from build123d import *

# Parameters (mm, degrees)
F1_DEPTH = 63.5
F0_W     = 25.4
F0_H     = 19.05
F2_DEPTH = 25.4
F3_DEPTH = 7.9375
F5_R     = 6.35


with BuildPart() as f1:
    # F0 (on Front) → F1 (new body, symmetric)
    with BuildSketch(Plane.XZ):
        Polygon((-41.275, 9.525), (-41.275, -9.525), (41.275, -9.525), (41.275, 9.525), (22.225, 9.525), align=None)
    extrude(amount=F1_DEPTH, both=True)

    # F0 (on Front) → F2 (join, symmetric)
    with BuildSketch(Plane.XZ):
        with BuildLine():
            Line((22.225, 9.525), (41.275, 9.525))
            Line((41.275, 9.525), (41.275, 27.0002))
            ThreePointArc((41.275, 27.0002), (45.9246798487, 38.2255201513), (57.15, 42.8752))
            Line((57.15, 42.8752), (60.325, 42.8752))
            Line((60.325, 42.8752), (60.325, 61.9252))
            Line((60.325, 61.9252), (57.15, 61.9252))
            ThreePointArc((57.15, 61.9252), (32.4542956671, 51.6959043329), (22.225, 27.0002))
            Line((22.225, 27.0002), (22.225, 9.525))
        make_face()
        with Locations((73.025, 52.4002)):
            Rectangle(F0_W, F0_H)
    extrude(amount=F2_DEPTH, both=True)

    # F0 (on Front) → F3 (join, symmetric)
    with BuildSketch(Plane.XZ):
        with BuildLine():
            add(Edge.make_bspline(
                [(-41.275, 9.525), (-41.1149449646, 36.8104875088), (6.9761793129, 62.6372024417), (57.15, 61.9252)],
                knots=[0, 0, 0, 0, 111.5045361635, 111.5045361635, 111.5045361635, 111.5045361635], degree=3))
            Line((-41.275, 9.525), (22.225, 9.525))
            Line((22.225, 9.525), (22.225, 27.0002))
            ThreePointArc((22.225, 27.0002), (32.4542956671, 51.6959043329), (57.15, 61.9252))
        make_face()
    extrude(amount=F3_DEPTH, both=True)

    # F0 (on Front) → F4 (revolve)
    with BuildSketch(Plane.XZ):
        Polygon((85.725, 66.675), (85.725, 61.9252), (85.725, 42.8752), (85.725, 38.1), (111.125, 38.1), (111.125, 66.675), align=None)
    revolve(axis=Axis((85.725, 0, 52.3875), (0, 0, 1)))

    # F5
    f5_edges = [f1.edges().sort_by_distance(p)[0] for p in [
        (-41.275, -63.5, 0),
        (41.275, -63.5, 0),
        (41.275, 63.5, 0),
        (41.275, 0, -9.525),
        (-41.275, 63.5, 0),
    ]]
    fillet(f5_edges, radius=F5_R)


solid = f1.part
Input: part model. Units: mm. Frame: model coordinates. A direction names the side the tool comes from. Round coordinates to 2 decimals unless told otherwise and drop trailing zeros. Order: outer loops, then holes, each group sorted by start corner. A loop starts at its lowest first (then second) coordinate and runs counter-clockwise, first axis right, second up. Notation, with made-up numbers: (68.25, 17.5) - (112.25, 17.5) arc R27 ccw to (112.25, 40.5) - close; hole circle Ø2 at (50, 47.5). An arc over 180 degrees is marked (long way). Use a Markdown table: item, result.
1. Mould query, pull axis X, two halves, no side actions, for faces 1 (the face through (-41.275, -1, 0)), 2 (the face through (86, 0, 38.1)), 3 (the face through (60, 2, 42.875)). Classes: +X half, -X half, draft (parallel to the pull), parting line (faces both ways), or undercut.
Evaluation:
| item | result |
|---|---|
| face 1 | -X half |
| face 2 | draft |
| face 3 | undercut |
2. Access query for faces 4 (the face through (46, -25.4, 42)), 5 (the face through (60, -2, 61.925)), 6 (the face through (22.225, 17, 18)), 7 (the face through (22.225, -17, 18)). Directions: +Z, -Z, +X, -X, +Y, -Y. A direction counts if a zero-diameter tool reaches every point of the face in a straight line with its end or side. Return the directions, or none.
Evaluation:
| item | result |
|---|---|
| face 4 | +Z, +X, -X, -Y |
| face 5 | +Z, -X |
| face 6 | +Z, -X, +Y |
| face 7 | +Z, -X, -Y |
3. First-contact query: pin 1 (6 mm diameter, centred on x = 22.5, y = -21, fed in from +Z); pin 2 (1 mm diameter, centred on y = 6, z = 15.5, fed in from -X); pin 3 (8.5 mm diameter, centred on y = -18.5, z = 16.5, fed in from -X) (3 decimals). Flat tips, straight axial feed; report the tip coordinate or a pass-through.
Evaluation:
| item | result |
|---|---|
| pin 1 | z = 41.77 |
| pin 2 | x = -40.61 |
| pin 3 | x = 22.225 |
4. Section B-B on x = 78.5. Return the cut outline in (y, z) (3 decimals), then the cut area to 3 significant figures.
Evaluation:
| item | result |
|---|---|
| outline | (-25.4, 42.875) - (-24.351, 42.875) - (-24.351, 38.1) - (24.351, 38.1) - (24.351, 42.875) - (25.4, 42.875) - (25.4, 61.925) - (24.351, 61.925) - (24.351, 66.675) - (-24.351, 66.675) - (-24.351, 61.925) - (-25.4, 61.925) - close |
| area | 1,430 mm^2 |
5. Material intervals for probe 1 along X at (y, z) = (-32, 3.5) (3 decimals); probe 2 along Z at (x, y) = (97, 5.5) (3 decimals); probe 3 along Z at (x, y) = (33.5, -35) (3 decimals), sorted ascending.
Evaluation:
| item | result |
|---|---|
| probe 1 | -41.275 to 41.275 |
| probe 2 | 38.1 to 66.675 |
| probe 3 | -9.525 to 9.525 |
6. Section A-A on z = 7.5. Return the cut outline in (x, y) (3 decimals), then the cut area to 3 significant figures.
Evaluation:
| item | result |
|---|---|
| outline | (-41.275, -57.15) arc R6.35 ccw to (-34.925, -63.5) - (34.925, -63.5) arc R6.35 ccw to (41.275, -57.15) - (41.275, 57.15) arc R6.35 ccw to (34.925, 63.5) - (-34.925, 63.5) arc R6.35 ccw to (-41.275, 57.15) - close |
| area | 10,400 mm^2 |
7. Section C-C on y = -33. Return the cut outline in (x, z) (3 decimals).
Evaluation:
| item | result |
|---|---|
| outline | (-41.275, -9.525) - (34.925, -9.525) arc R6.35 ccw to (41.275, -3.175) - (41.275, 9.525) - (-41.275, 9.525) - close |
